Can you work these out from the model? Positions are in its coordinate system, mm. Face numbers are marked on the shaded views. A direction names the side the tool comes from. Coordinates: 2 decimals unless noted, no trailing zeros. Loops run counter-clockwise (first coordinate to the right, second up) from the corner with the lowest first, then second, coordinate; pieces in that order, holes last. Notation, with made-up numbers: (52.25, -27) - (58.25, -27) arc R19 ccw to (58.25, -4) - close; hole circle Ø1 at (88.5, 10.25). An arc over 180 degrees is marked (long way). Put each result on its own line as item: value. Start each with the question number.
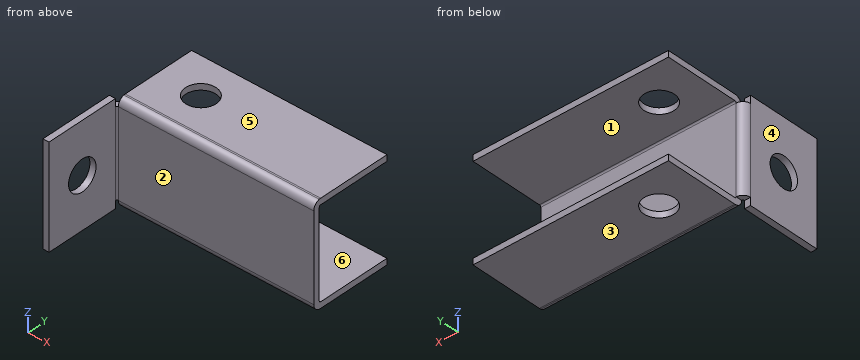
from build123d import *

# Parameters (mm, degrees)
SKETCH1_W                    = 100
SKETCH1_H                    = 50
BASE_FLANGE1_DEPTH           = 3
EDGE_FLANGE1_STRIP_W         = 13.4732
EDGE_FLANGE1_STRIP_H         = 3
EDGE_FLANGE1_STRIP_CUT_DEPTH = 50
EDGE_FLANGE1_DEPTH           = 50
EDGE_FLANGE2_START           = -50
EDGE_FLANGE2_DEPTH           = 100
EDGE_FLANGE2_2_DEPTH         = 3.7366
EDGE_FLANGE2_START_2         = -46.2634
EDGE_FLANGE2_3_DEPTH         = 96.2634
SKETCH15_R                   = 7.5
CUT_EXTRUDE1_DEPTH           = 82.240384046
CUT_EXTRUDE2_REACH           = 112.567
SKETCH16_R                   = 7.5


# Read off the part's stored shape, not the designer's step: Edge-Flange2
# Sheet-metal steps are written as plain solids
with BuildPart() as part:
    # Sketch1 → Base-Flange1 (new body)
    with BuildSketch(Plane(origin=(0, 0, 0), x_dir=(1, 0, 0), z_dir=(0, 1, 0))):
        Rectangle(SKETCH1_W, SKETCH1_H)
    extrude(amount=-BASE_FLANGE1_DEPTH)

    # Edge-Flange1 strip (across the edge) → Edge-Flange1 strip cut (cut)
    with BuildSketch(Plane(origin=(-50, -3, 25), x_dir=(1, 0, 0), z_dir=(0, 0, -1))):
        with Locations((-3, -1.5)):
            Rectangle(EDGE_FLANGE1_STRIP_W, EDGE_FLANGE1_STRIP_H)
    extrude(amount=EDGE_FLANGE1_STRIP_CUT_DEPTH, mode=Mode.SUBTRACT)

    # Edge-Flange1 section (across the edge) → Edge-Flange1 (add)
    with BuildSketch(Plane(origin=(-50, -3, 25), x_dir=(1, 0, 0), z_dir=(0, 0, -1))):
        with BuildLine():
            Line((0, 0.7366), (0, 37))
            Line((0, 37), (3, 37))
            Line((3, 37), (3, 0.7366))
            ThreePointArc((3, 0.7366), (3.215745145, 0.215745145), (3.7366, 0))
            Line((3.7366, 0), (3.7366, -3))
            ThreePointArc((3.7366, -3), (1.094424801, -1.905575199), (0, 0.7366))
        make_face()
    extrude(amount=EDGE_FLANGE1_DEPTH)

    # Edge-Flange2 outline → Edge-Flange2 (cut)
    with BuildSketch(Plane.YZ.offset(EDGE_FLANGE2_START)):
        with BuildLine():
            Line((-3, -21.2634), (-3.7366, -21.2634))
            Line((-3.7366, -21.2634), (-3.7366, -25))
            Line((-3.7366, -25), (0, -25))
            Line((0, -25), (0, -24.926677222))
            ThreePointArc((0, -24.926677222), (-2.154295979, -23.630867001), (-3, -21.2634))
        make_face()
        with BuildLine():
            Line((0, 25), (-3.7366, 25))
            Line((-3.7366, 25), (-3.7366, 21.2634))
            Line((-3.7366, 21.2634), (-3, 21.2634))
            ThreePointArc((-3, 21.2634), (-2.154295979, 23.630867001), (0, 24.926677222))
            Line((0, 24.926677222), (0, 25))
        make_face()
    extrude(amount=EDGE_FLANGE2_DEPTH, mode=Mode.SUBTRACT)

    # Edge-Flange2 2 outline → Edge-Flange2 2 (cut)
    with BuildSketch(Plane.YZ.offset(EDGE_FLANGE2_START)):
        with BuildLine():
            Line((0, -21.2634), (-3, -21.2634))
            ThreePointArc((-3, -21.2634), (-2.154295979, -23.630867001), (0, -24.926677222))
            Line((0, -24.926677222), (0, -21.2634))
        make_face()
        with BuildLine():
            ThreePointArc((0, 24.926677222), (-2.154295979, 23.630867001), (-3, 21.2634))
            Line((-3, 21.2634), (0, 21.2634))
            Line((0, 21.2634), (0, 24.926677222))
        make_face()
    extrude(amount=EDGE_FLANGE2_2_DEPTH, mode=Mode.SUBTRACT)

    # Edge-Flange2 3 outline → Edge-Flange2 3 (add)
    with BuildSketch(Plane.YZ.offset(EDGE_FLANGE2_START_2)):
        with BuildLine():
            ThreePointArc((0.7366, -22), (0.215745145, -21.784254855), (0, -21.2634))
            Line((0, -21.2634), (0, -24.926677222))
            ThreePointArc((0, -24.926677222), (0.36647982, -24.981624121), (0.7366, -25))
            Line((0.7366, -25), (37, -25))
            Line((37, -25), (37, -22))
            Line((37, -22), (0.7366, -22))
        make_face()
        with BuildLine():
            Line((0, 24.926677222), (0, 21.2634))
            ThreePointArc((0, 21.2634), (0.215745145, 21.784254855), (0.7366, 22))
            Line((0.7366, 22), (37, 22))
            Line((37, 22), (37, 25))
            Line((37, 25), (0.7366, 25))
            ThreePointArc((0.7366, 25), (0.36647982, 24.981624121), (0, 24.926677222))
        make_face()
    extrude(amount=EDGE_FLANGE2_3_DEPTH)

    # Sketch15 → Cut-Extrude1 (cut, through all)
    with BuildSketch(Plane.XY.offset(25)):
        with Locations((-25, 18.5)):
            Circle(SKETCH15_R)
    extrude(amount=-CUT_EXTRUDE1_DEPTH, mode=Mode.SUBTRACT)

    # Sketch16 → Cut-Extrude2 (cut, up to next)
    with BuildSketch(Plane.ZY.offset(50), mode=Mode.PRIVATE) as cut_extrude2_sk1:
        with Locations(Location((0, -21.8683, 0), (0, 0, 270))):
            Circle(SKETCH16_R)
    cut_extrude2_tool1 = extrude(cut_extrude2_sk1.sketch, amount=-CUT_EXTRUDE2_REACH, mode=Mode.PRIVATE) & part.part
    add(cut_extrude2_tool1.solids().sort_by_distance((-50, -21.8683, 0))[0], mode=Mode.SUBTRACT)


solid = part.part
Q1. I want a section at B-B on y = 18.5. List the corners of the cut face in (x, z) for me, and give its area (3 significant figures).
Q2. I want a section at A-A on x = -25. List the corners of the cut face in (y, z) for me.
Q3. We'd pull the mould along Z, two halves only. Please class the marked faces 4, 5 and 6: released by +Z, released by -Z, zero draft, split by the parting line, or undercut.
Q4. Please list where these lines run through material, in increasing order: line 1 along Z through (x, y) = (-11, 20.5); line 2 along X through (y, z) = (18, 23); line 3 along X through (y, z) = (-32.5, 11.5). Write a range as [from, to].
Q5. Will these pins go through, and if not, where does the flat tip stop? pin 1 (8 mm diameter, centred on x = 37, z = -12, fed in from +Y); pin 2 (3 mm diameter, centred on y = 18.5, z = 23, fed in from -X); pin 3 (3 mm diameter, centred on x = -1, y = -1, fed in from +Z).
Q6. I want a section at D-D on z = 14. List the corners of the cut face in (x, y) for me, and give its area (3 significant figures).
Q7. On a 3-axis mill with a long thin cutter (end or side, diameter ignored), from which of +Z, -Z, +X, -X, +Y, -Y can I reach the whole of each face in a straight line? I mean the marked faces 1, 2 and 3. Say none if no direction works.
Q8. I want a section at C-C on z = 1.5. List the corners of the cut face in (x, y) for me.
Calculated:
1. outline: (-46.26, -25) - (-32.5, -25) - (-32.5, -22) - (-46.26, -22) - close; (-46.26, 22) - (-32.5, 22) - (-32.5, 25) - (-46.26, 25) - close; (-17.5, -25) - (50, -25) - (50, -22) - (-17.5, -22) - close; (-17.5, 22) - (50, 22) - (50, 25) - (-17.5, 25) - close
1. area: 488 mm2
2. outline: (-3, -21.26) arc R3.74 ccw to (0.74, -25) - (11, -25) - (11, -22) - (0.74, -22) arc R0.74 cw to (0, -21.26) - (0, 21.26) arc R0.74 cw to (0.74, 22) - (11, 22) - (11, 25) - (0.74, 25) arc R3.74 ccw to (-3, 21.26) - close; (26, -25) - (37, -25) - (37, -22) - (26, -22) - close; (26, 22) - (37, 22) - (37, 25) - (26, 25) - close
3. face 4: zero draft
3. face 5: released by +Z
3. face 6: undercut
4. line 1: [-25, -22], [22, 25]
4. line 2: [-46.26, -32.48], [-17.52, 50]
4. line 3: [-50, -47]
5. pin 1: y = 0
5. pin 2: x = -46.26
5. pin 3: z = 24.99
6. outline: (-50, -40) - (-47, -40) - (-47, -3.74) arc R0.74 cw to (-46.26, -3) - (50, -3) - (50, 0) - (-46.26, 0) arc R3.74 ccw to (-50, -3.74) - close
6. area: 408 mm2
7. face 1: +X, -X, +Y
7. face 2: +Z, -Z, +X, -Y
7. face 3: -Z, +X, -X, +Y, -Y
8. outline: (-50, -40) - (-47, -40) - (-47, -29.22) - (-50, -29.22) - close; (-50, -14.52) - (-47, -14.52) - (-47, -3.74) arc R0.74 cw to (-46.26, -3) - (50, -3) - (50, 0) - (-46.26, 0) arc R3.74 ccw to (-50, -3.74) - close
